Autodesk Inventor part; units mm, degrees
ref_plane "YZ Plane" through (0, 0, 0) normal (1, 0, 0) x (0, 1, 0)
ref_plane "XZ Plane" through (0, 0, 0) normal (0, 1, 0) x (-1, 0, 0)
ref_plane "XY Plane" through (0, 0, 0) normal (0, 0, 1) x (1, 0, 0)
sketch "Sketch1" plane through (0, 0, 0) normal (0, 1, 0) x (-1, 0, 0)
  line L0 (-25, 20) -> (25, 20)
  line L1 (25, 20) -> (25, -20)
  line L2 (25, -20) -> (-25, -20)
  line L3 (-25, -20) -> (-25, 20)
  line L4 (-25, 20) -> (25, -20) construction
  line L5 (25, 20) -> (-25, -20) construction
  point P0 (0, 0)
  dimension "length" = 50
  dimension "width" = 40
extrude "Extrusion1" add sketch "Sketch1" along normal blind 1.5875
hole "Hole1" at (22.5, 1.5875, 17.5) direction (0, -1, 0) diameter 2.2 end through all
pattern_linear "Rectangular Pattern2" count 2 spacing 45 along (-1, 0, 0) count 2 spacing 35 along (0, 0, -1) of "Hole1"
sketch "Sketch2" plane through (0, 1.5875, 0) normal (0, 1, 0) x (1, 0, 0)
  line L0 (25, -20) -> (25, 20)
  line L1 (5, 0) -> (14.1924, -9.1924) construction
  line L2 (5, 0) -> (18, 0) construction
  line L3 (25, 20) -> (-25, 20) construction
  line L4 (5, 0) -> (8.3646, -12.557) construction
  line L5 (5, 0) -> (1.6354, -12.557) construction
  line L6 (5, 0) -> (-4.1924, -9.1924) construction
  line L7 (5, 0) -> (-7.557, -3.3646) construction
  line L8 (5, 0) -> (-7.557, 3.3646) construction
  line L9 (5, 0) -> (-4.1924, 9.1924) construction
  line L10 (5, 0) -> (1.6354, 12.557) construction
  line L11 (5, 0) -> (8.3646, 12.557) construction
  line L12 (5, 0) -> (14.1924, 9.1924) construction
  line L13 (14.1924, -9.1924) -> (12.1604, -7.1604) construction
  circle A0 centre (12.1604, -7.1604) radius 0.305
  circle A1 centre (16.2244, -11.2244) radius 0.305
  circle A2 centre (6.3326, -10.525) radius 0.305
  circle A3 centre (10.3966, -14.589) radius 0.305
  circle A4 centre (-0.3966, -10.525) radius 0.305
  circle A5 centre (3.6674, -14.589) radius 0.305
  circle A6 centre (-6.2244, -7.1604) radius 0.305
  circle A7 centre (-2.1604, -11.2244) radius 0.305
  circle A8 centre (-9.589, -1.3326) radius 0.305
  circle A9 centre (-5.525, -5.3966) radius 0.305
  circle A10 centre (-9.589, 5.3966) radius 0.305
  circle A11 centre (-5.525, 1.3326) radius 0.305
  circle A12 centre (-6.2244, 11.2244) radius 0.305
  circle A13 centre (-2.1604, 7.1604) radius 0.305
  circle A14 centre (-0.3966, 14.589) radius 0.305
  circle A15 centre (3.6674, 10.525) radius 0.305
  circle A16 centre (6.3326, 14.589) radius 0.305
  circle A17 centre (10.3966, 10.525) radius 0.305
  circle A18 centre (12.1604, 11.2244) radius 0.305
  circle A19 centre (16.2244, 7.1604) radius 0.305
  point P0 (0, 0)
  dimension "d14" = 20
  dimension "d15" = 13
  dimension "d16" = 45
  dimension "d17" = 20
  dimension "d20" = 270
  dimension "d22" = 2.032
  dimension "d23" = 2.032
  dimension "d24" = 0.61
  dimension "d27" = 360
  dimension "d33" = 0.61
  dimension "d38" = 0.61
  dimension "d43" = 0.61
  dimension "d48" = 0.61
  dimension "d53" = 0.61
  dimension "d58" = 0.61
  dimension "d63" = 0.61
  dimension "d68" = 0.61
  dimension "d73" = 0.61
hole "Hole2" at (16.2244, 1.5875, 11.2244) at (12.1604, 1.5875, 7.1604) at (16.2244, 1.5875, -7.1604) at (10.3966, 1.5875, 14.589) at (6.3326, 1.5875, 10.525) at (3.6674, 1.5875, 14.589) at (-0.3966, 1.5875, 10.525) at (-2.1604, 1.5875, 11.2244) at (-5.525, 1.5875, 5.3966) at (-6.2244, 1.5875, 7.1604) at (-9.589, 1.5875, 1.3326) at (-5.525, 1.5875, -1.3326) at (-9.589, 1.5875, -5.3966) at (-2.1604, 1.5875, -7.1604) at (-6.2244, 1.5875, -11.2244) at (-0.3966, 1.5875, -14.589) at (3.6674, 1.5875, -10.525) at (6.3326, 1.5875, -14.589) at (10.3966, 1.5875, -10.525) at (12.1604, 1.5875, -11.2244) direction (0, -1, 0) diameter 0.61 end through all
sketch "Sketch3" plane through (0, 1.5875, 0) normal (0, 1, 0) x (1, 0, 0)
  line L0 (25, 20) -> (-25, 20)
  line L1 (25, -20) -> (25, 20)
  line L2 (5, 0) -> (5, -5.7) construction
  line L3 (5.4, -6.6) -> (4.6, -6.6)
  line L4 (4.6, -6.6) -> (4.6, -4.8)
  line L5 (4.6, -4.8) -> (5.4, -4.8)
  line L6 (5.4, -4.8) -> (5.4, -6.6)
  line L7 (5.4, -6.6) -> (4.6, -4.8) construction
  line L8 (4.6, -6.6) -> (5.4, -4.8) construction
  circle A0 centre (4.6, -5.7) radius 0.9
  circle A1 centre (5.4, -5.7) radius 0.9
  point P0 (0, 0)
  dimension "d81" = 20
  dimension "d82" = 20
  dimension "d83" = 5.7
  dimension "d86" = 0.8
  dimension "d87" = 1.8
extrude "Cut1" cut sketch "Sketch3" against normal blind 3.048
mirror "Mirror3" about plane through (0, 0, 0) normal (0, 0, 1) of "Cut1"
hole "Hole3" at (5, 1.5875, 0.0102) direction (0, -1, 0) diameter 6.35 depth 3.048 tip angle 118
sketch "Sketch5" plane through (0, 1.5875, 0) normal (0, 1, 0) x (1, 0, 0)
  circle A0 centre (5, -0.0102) radius 3.175
  line L0 (-25, 20) -> (-25, -20)
  point P0 (0, 0)
  point P1 (-20.5, -12.5102)
  point P2 (-18.468, -14.5422)
  point P3 (-22.532, -10.4782)
  dimension "d100" = 25.5
  dimension "d101" = 12.5
  dimension "d115" = 2.032
  dimension "d116" = 2.032
  dimension "d117" = 2.032
  dimension "d118" = 2.032
hole "Hole4" at (-18.468, 1.5875, 14.5422) at (-22.532, 1.5875, 10.4782) direction (0, -1, 0) diameter 0.6096 end through all
pattern_linear "Rectangular Pattern1" count 6 spacing 5 along (0, 0, -1) of "Hole4"
equation "\"d5\" = holeOffset"
equation "\"d131\" = length - 2 * holeOffset"
equation "\"d134\" = width - 2 * holeOffset"
equation "\"d88\" = Thickness"
equation "\"d97\" = Thickness"
equation "\"d124\" = Thickness"
equation "\"BendRadius\" = Thickness"
equation "\"BendReliefWidth\" = Thickness"
equation "\"BendReliefDepth\" = 0.5 * Thickness"
equation "\"CornerReliefSize\" = 4 * Thickness"
equation "\"MinimumRemnant\" = 2 * Thickness"
equation "\"TransitionRadius\" = BendRadius"
equation "\"JacobiRadiusSize\" = Thickness"
equation "\"GapSize\" = Thickness"
properties part number "pcb rotary control"
Design review of the part built by this model. Coordinates are the model's own, in mm. A direction names the side the tool comes from. Give positions to 0.01 mm unless a question says otherwise; leave off trailing zeros. Order: outer loops, then holes, each group sorted by start corner. A loop starts at its lowest first (then second) coordinate and runs counter-clockwise, first axis right, second up. Notation, with made-up numbers: (61.25, 15.25) -> (67.25, 15.25) arc R25 cw to (67.25, 42.25) -> close; hole circle Ø11 at (71.5, -26). An arc over 180 degrees is marked (long way). Write item = value, one per line. Start each with the question number.
(1) We need section A-A on z = 17.5. Write out the cut boundary in (x, y).
(2) To check wall thickness, follow line 1 along X through (y, z) = (0.7, -17.5); line 2 along X through (y, z) = (1.3, -1.5); line 3 along Z through (x, y) = (4.5, 0.2). State the ranges of each line that lie inside material, in increasing order.
(3) Mouldability with a two-part tool opening along X and no side actions: class faces 3 (the face through (0, 0, 0)), 4 (the face through (6.3, 0.8, 5.7)), 5 (the face through (-25, 1, 0)), 6 (the face through (7.817, 0.783, 1.475)) as +X half, -X half, draft (parallel to the pull), parting line (faces both ways), or undercut.
(4) We need section B-B on y = 0.8. State how many separate pieces and enclosed holes the cut face has, plus the area to 3 significant figures.
(5) For faces 1 (the face through (3.7, 0.8, 5.7)), 2 (the face through (0, 1.588, 0)), list the 3-axis set-ups (+Z, -Z, +X, -X, +Y, -Y) from which the entire face can be reached by the end or side of a thin tool; tool diameter is ignored.
Numbers:
q1.outline = (-25, 0) -> (-23.6, 0) -> (-23.6, 1.59) -> (-25, 1.59) -> close; (-21.4, 0) -> (21.4, 0) -> (21.4, 1.59) -> (-21.4, 1.59) -> close; (23.6, 0) -> (25, 0) -> (25, 1.59) -> (23.6, 1.59) -> close
q2.line_1 = -25 to -23.6, -21.4 to 21.4, 23.6 to 25
q2.line_2 = -25 to -5.78, -5.27 to 2.21, 7.79 to 25
q2.line_3 = -20 to -6.59, -4.81 to -3.13, 3.15 to 4.81, 6.59 to 20
q3.face_3 = draft
q3.face_4 = undercut
q3.face_5 = -X half
q3.face_6 = undercut
q4.separate_pieces = 1
q4.enclosed_holes = 39
q4.area = 1,940 mm^2
q5.face_1 = +Y, -Y
q5.face_2 = +Z, -Z, +X, -X, +Y
